from build123d import *

# Parameters (mm, degrees)
F0_W     = 29
F0_H     = 29
F1_DEPTH = 11
F2_R     = 2.6
F3_DEPTH = 11.001
F4_W     = 0.8
F4_H     = 6.3
F5_DEPTH = 13.7


with BuildPart() as f1:
    # F0 (on Top) → F1 (new body)
    with BuildSketch(Plane.XY):
        Rectangle(F0_W, F0_H)
    extrude(amount=F1_DEPTH)

    # F2 (on face) → F3 (cut, through all)
    with BuildSketch(Plane.XY.offset(11)):
        Circle(F2_R)
    extrude(amount=-F3_DEPTH, mode=Mode.SUBTRACT)

    # F4 (on face) → F5 (join)
    with BuildSketch(Plane.XY.offset(11)):
        with Locations((9.4, 8.4)):
            Rectangle(F4_W, F4_H)
        with Locations((9.4, -6.6)):
            Rectangle(F4_W, F4_H)
        with Locations((-8.6, 8.4)):
            Rectangle(F4_W, F4_H)
        with Locations((-8.6, -6.6)):
            Rectangle(F4_W, F4_H)
    extrude(amount=F5_DEPTH)


solid = f1.part
Input: part model. Units: mm. Frame: model coordinates. A direction names the side the tool comes from. Coordinates: 2 decimals unless noted, no trailing zeros. Order: outer loops, then holes, each group sorted by start corner. A loop starts at its lowest first (then second) coordinate and runs counter-clockwise, first axis right, second up. Notation, with made-up numbers: M 33,58.25 L 46,58.25 A34 cw 46,88.25 Z; hole C 54,1 d7. An arc over 180 degrees is marked long. Answer in a Markdown table with one row per item.
(1) Material intervals for line 1 (X direction, y = -8.25, z = 17.75); line 2 (Y direction, x = 0, z = 8.25); line 3 (Z direction, x = -12.5, y = 7.25), sorted ascending. Write a range as [from, to].
Numbers:
| item | result |
|---|---|
| line 1 | x = [-9, -8.2], [9, 9.8] |
| line 2 | y = [-14.5, -2.6], [2.6, 14.5] |
| line 3 | z = [0, 11] |
(2) Section query D-D, the plane z = 2. Output: boundary loops of the cut face in (x, y), plus the area to 3 significant figures.
Numbers:
| item | result |
|---|---|
| outline | M -14.5,-14.5 L 14.5,-14.5 L 14.5,14.5 L -14.5,14.5 Z; hole C 0,0 d5.2 |
| area | 820 mm^2 |
(3) Section query A-A, the plane z = 16. Output: boundary loops of the cut face in (x, y), plus the area to 3 significant figures.
Numbers:
| item | result |
|---|---|
| outline | M -9,-9.75 L -8.2,-9.75 L -8.2,-3.45 L -9,-3.45 Z; M -9,5.25 L -8.2,5.25 L -8.2,11.55 L -9,11.55 Z; M 9,-9.75 L 9.8,-9.75 L 9.8,-3.45 L 9,-3.45 Z; M 9,5.25 L 9.8,5.25 L 9.8,11.55 L 9,11.55 Z |
| area | 20.2 mm^2 |
(4) Access query for faces 1 (the flat face through (-9, 8, 18)), 2 (the flat face through (9.8, -7, 18)), 3 (the flat face through (9.4, -3.45, 17.8)), 4 (the flat face through (9.4, -9.75, 17.8)), 5 (the flat face through (9.4, 11.55, 17.8)). Directions: +Z, -Z, +X, -X, +Y, -Y. A direction counts if a zero-diameter tool reaches every point of the face in a straight line with its end or side. Return the directions, or none.
Numbers:
| item | result |
|---|---|
| face 1 | +Z, -X, +Y, -Y |
| face 2 | +Z, +X, +Y, -Y |
| face 3 | +Z, +X, -X |
| face 4 | +Z, +X, -X, -Y |
| face 5 | +Z, +X, -X, +Y |
(5) Section query B-B, the plane y = 0. Output: boundary loops of the cut face in (x, z), plus the area to 3 significant figures.
Numbers:
| item | result |
|---|---|
| outline | M -14.5,0 L -2.6,0 L -2.6,11 L -14.5,11 Z; M 2.6,0 L 14.5,0 L 14.5,11 L 2.6,11 Z |
| area | 262 mm^2 |
(6) Contact query for flat-ended pins moving along their axis: pin 1 Ø1.9 at (y, z) = (-5, 15) entering from +X; pin 2 Ø0.9 at (x, z) = (-9, 18.5) entering from +Y; pin 3 Ø0.6 at (x, z) = (-8.5, 19) entering from -Y. Output: stop coordinate, or through.
Numbers:
| item | result |
|---|---|
| pin 1 | stops at x = 9.8 |
| pin 2 | stops at y = 11.55 |
| pin 3 | stops at y = -9.75 |
(7) Draft query along X for faces 6 (the flat face through (0, 14.5, 5)), 7 (the flat face through (-9, -7, 18)), 8 (the flat face through (9, -7, 18)), 9 (the flat face through (-8.2, -7, 18)). Return one class per face: pulls with the +X half, pulls with the -X half, needs draft (parallel to the pull), parting line crosses it, or undercut.
Numbers:
| item | result |
|---|---|
| face 6 | needs draft |
| face 7 | pulls with the -X half |
| face 8 | undercut |
| face 9 | undercut |
